Answer from the drawing. Dimensions are ordinates in mm from the lowest x, y and z of the part. A direction names the side the tool comes from. Coordinates: 2 decimals unless noted, no trailing zeros. Order: outer loops, then holes, each group sorted by start corner. A loop starts at its lowest first (then second) coordinate and runs counter-clockwise, first axis right, second up. Notation, with made-up numbers: M 89,60 L 147,60 A36 ccw 147,94 Z; hole C 11.5,79.5 d9. An arc over 180 degrees is marked long. Use a Markdown table: item, result.
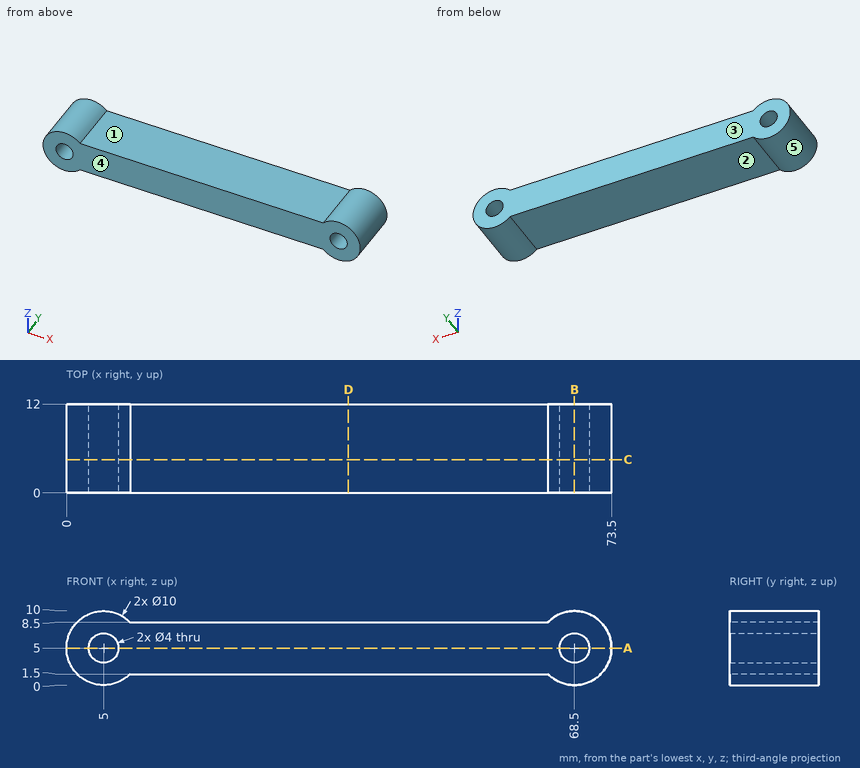
(1) A cutting plane is placed at D-D (x = 38). Determine the outline of the cut face in (y, z), then the cut area to 3 significant figures.
Conclusion:
| item | result |
|---|---|
| outline | M 0,1.5 L 12,1.5 L 12,8.5 L 0,8.5 Z |
| area | 84.0 mm2 |
(2) Which of the six approach directions +Z, -Z, +X, -X, +Y, -Y give full straight-line access (tool end or side, diameter ignored) to the marked faces 1, 2 and 3?
Conclusion:
| item | result |
|---|---|
| face 1 | +Z, +Y, -Y |
| face 2 | -Z, +Y, -Y |
| face 3 | +Z, -Z, +X, -X, +Y |
(3) A cutting plane is placed at B-B (x = 68.5). Determine the outline of the cut face in (y, z), then the cut area to 3 significant figures.
Conclusion:
| item | result |
|---|---|
| outline | M 0,0 L 12,0 L 12,3 L 0,3 Z; M 0,7 L 12,7 L 12,10 L 0,10 Z |
| area | 72.0 mm2 |
(4) Straight lines are drawn through the part: L1, parallel to X at y = 4.75, z = 5; L2, parallel to Z at x = 68.5, y = 7.5; L3, parallel to X at y = 6.5, z = 4.5. For each, find the intervals that lie inside material, in ascending order.
Conclusion:
| item | result |
|---|---|
| L1 | 0 to 3, 7 to 66.5, 70.5 to 73.5 |
| L2 | 0 to 3, 7 to 10 |
| L3 | 0.03 to 3.06, 6.94 to 66.56, 70.44 to 73.47 |
(5) A cutting plane is placed at A-A (z = 5). Determine the outline of the cut face in (x, y).
Conclusion:
| item | result |
|---|---|
| outline | M 0,0 L 3,0 L 3,12 L 0,12 Z; M 7,0 L 66.5,0 L 66.5,12 L 7,12 Z; M 70.5,0 L 73.5,0 L 73.5,12 L 70.5,12 Z |
(6) A cutting plane is placed at C-C (y = 4.5). Determine the outline of the cut face in (x, z).
Conclusion:
| item | result |
|---|---|
| outline | M 8.57,1.5 L 64.93,1.5 A5 ccw long 64.93,8.5 L 8.57,8.5 A5 ccw long Z; hole C 5,5 d4; hole C 68.5,5 d4 |
(7) Determine the mould class of the marked faces 4 and 5 for opening direction X: pulls with the +X half, pulls with the -X half, needs draft (parallel to the pull), parting line crosses it, or undercut.
Conclusion:
| item | result |
|---|---|
| face 4 | needs draft |
| face 5 | undercut |
(8) Given P1, Ø5, axis at x = 57, y = 5.5, coming from the -Z side; P2, Ø1, axis at x = 19, y = 10, coming from the +Z side; P3, Ø2, axis at y = 8, z = 7, coming from the -X side, each flat-ended and moving along its own axis, determine where each tip first touches the part or whether it passes through.
Conclusion:
| item | result |
|---|---|
| P1 | z = 1.5 |
| P2 | z = 8.5 |
| P3 | x = 0.1 |
